Input: part model. Units: mm. Frame: model coordinates. A direction names the side the tool comes from. Round coordinates to 2 decimals unless told otherwise and drop trailing zeros. Loops run counter-clockwise (first coordinate to the right, second up) from the corner with the lowest first, then second, coordinate; pieces in that order, holes last. Notation, with made-up numbers: (44.25, 55) -> (55.25, 55) arc R8 ccw to (55.25, 69) -> close; hole circle Ø7 at (12.5, -0.5). An arc over 180 degrees is marked (long way). Answer in a Markdown table with one row per item. Add a question column.
Q1. Section D-D, the plane z = 2.75. Output: boundary loops of the cut face in (x, y), and give its area (3 significant figures).
Q2. Pin query (flat end, axial travel): pin 1 (5 mm diameter, centred on y = -7, z = 2.5, fed in from +X); pin 2 (1 mm diameter, centred on x = -5.5, y = -3, fed in from +Z); pin 3 (10 mm diameter, centred on x = 6, y = -4.5, fed in from -Z); pin 4 (0.5 mm diameter, centred on x = -5, z = 6.5, fed in from -Y). Return the tip coordinate at first contact, or that it passes through.
Q3. Section A-A, the plane z = 6.5. Output: boundary loops of the cut face in (x, y), and give its area (3 significant figures).
Q4. Ray query, L1, parallel to Y at x = 0, z = 11.1; L2, parallel to Y at x = 0, z = 10.25; L3, parallel to Y at x = 0, z = 11.75. Return the intervals inside material, ascending. Write a range as from..to.
Q5. Section B-B, the plane x = 0. Give the number of separate pieces and of enclosed holes in the cut face, and give its area (3 significant figures).
Q6. Reachability of faces 1 (the face through (-1, 8, 10.5)), 2 (the face through (0, 0, 11)), 3 (the face through (5.15, -8.98, 11.7)) from +Z, -Z, +X, -X, +Y, -Y: full face, straight path, thin tool, end or side. Return the list, or none.
Q7. Section C-C, the plane y = 0. Output: boundary loops of the cut face in (x, z), and give its area (3 significant figures).
Q8. Mould query, pull axis Y, two halves, no side actions, for faces 4 (the face through (0.05, -14.55, 10.75)), 5 (the face through (5.225, 8.869, 11.699)), 6 (the face through (-4.175, 0, 7)). Classes: pulls with the +Y half, pulls with the -Y half, needs draft (parallel to the pull), parting line crosses it, or undercut.
```python
from build123d import *

# Parameters (mm, degrees)
SKETCH1_R           = 7.5
BOSS_EXTRUDE1_DEPTH = 10.5
FILLET1_R           = 1
SKETCH2_R           = 6
BOSS_EXTRUDE2_DEPTH = 2
SKETCH3_R           = 1.6
BOSS_EXTRUDE3_DEPTH = 1.5
FILLET2_R           = 1
SKETCH4_R           = 7
CUT_EXTRUDE1_DEPTH  = 8.34
SKETCH5_R           = 5.8
BOSS_EXTRUDE4_DEPTH = 7.34
CUT_EXTRUDE2_START  = -7.34
CUT_EXTRUDE2_DEPTH  = 7.34


with BuildPart() as part:
    # Sketch1 → Boss-Extrude1 (new body)
    with BuildSketch(Plane.XY):
        with Locations(Location((0, 0, 0), (0, 0, 180))):
            Circle(SKETCH1_R)
    extrude(amount=BOSS_EXTRUDE1_DEPTH)

    # Fillet1
    fillet1_edges = [part.edges().sort_by_distance(p)[0] for p in [
        (7.5, 0, 0),
    ]]
    fillet(fillet1_edges, radius=FILLET1_R)

    # Sketch2 → Boss-Extrude2 (add)
    with BuildSketch(Plane(origin=(0, 0, 0), x_dir=(-1, 0, 0), z_dir=(0, 0, -1))):
        with Locations(Location((0, 0, 0), (0, 0, 180))):
            Circle(SKETCH2_R)
    extrude(amount=BOSS_EXTRUDE2_DEPTH)

    # Sketch3 → Boss-Extrude3 (add)
    with BuildSketch(Plane.XY.offset(10.5)):
        with BuildLine():
            Line((-7.964864241, 5.177927928), (-2.89250333, 12.980405405))
            ThreePointArc((-2.89250333, 12.980405405), (0, 14.55), (2.89250333, 12.980405405))
            Line((2.89250333, 12.980405405), (7.964864241, 5.177927928))
            ThreePointArc((7.964864241, 5.177927928), (9.5, 0), (7.964864241, -5.177927928))
            Line((7.964864241, -5.177927928), (2.89250333, -12.980405405))
            ThreePointArc((2.89250333, -12.980405405), (0, -14.55), (-2.89250333, -12.980405405))
            Line((-2.89250333, -12.980405405), (-7.964864241, -5.177927928))
            ThreePointArc((-7.964864241, -5.177927928), (-9.5, 0), (-7.964864241, 5.177927928))
        make_face()
        with Locations((0, -11.1)):
            Circle(SKETCH3_R, mode=Mode.SUBTRACT)
        with Locations((0, 11.1)):
            Circle(SKETCH3_R, mode=Mode.SUBTRACT)
    extrude(amount=BOSS_EXTRUDE3_DEPTH)

    # Fillet2
    fillet2_edges = [part.edges().sort_by_distance(p)[0] for p in [
        (-9.5, 0, 12),
        (-5.428683785, -9.079166667, 12),
        (0, -14.55, 12),
        (5.428683785, -9.079166667, 12),
        (9.5, 0, 12),
        (5.428683785, 9.079166667, 12),
        (0, 14.55, 12),
        (-5.428683785, 9.079166667, 12),
    ]]
    fillet(fillet2_edges, radius=FILLET2_R)

    # Sketch4 → Cut-Extrude1 (cut)
    with BuildSketch(Plane.XY.offset(12)):
        Circle(SKETCH4_R)
    extrude(amount=-CUT_EXTRUDE1_DEPTH, mode=Mode.SUBTRACT)

    # Sketch5 → Boss-Extrude4 (add)
    with BuildSketch(Plane.XY.offset(3.66)):
        with Locations(Location((0, 0, 0), (0, 0, 180))):
            Circle(SKETCH5_R)
    extrude(amount=BOSS_EXTRUDE4_DEPTH)

    # Sketch6 → Cut-Extrude2 (cut)
    with BuildSketch(Plane.XY.offset(11).offset(CUT_EXTRUDE2_START)):
        with BuildLine():
            Line((-5.674504384, -1.2), (-4.174504384, -1.2))
            Line((-4.174504384, -1.2), (-4.174504384, 1.2))
            Line((-4.174504384, 1.2), (-5.674504384, 1.2))
            ThreePointArc((-5.674504384, 1.2), (-5.8, 0), (-5.674504384, -1.2))
        make_face()
    extrude(amount=CUT_EXTRUDE2_DEPTH, mode=Mode.SUBTRACT)


solid = part.part
```
Answer block:
| question | item | result |
|---|---|---|
| 1 | outline | circle Ø15 at (0, 0) |
| 1 | area | 177 mm^2 |
| 2 | pin 1 | x = 6 |
| 2 | pin 2 | z = 11 |
| 2 | pin 3 | z = -2 |
| 2 | pin 4 | y = -5.8 |
| 3 | outline | circle Ø15 at (0, 0); (-5.67, -1.2) arc R5.8 ccw (long way) to (-5.67, 1.2) -> (-4.17, 1.2) -> (-4.17, -1.2) -> close; hole circle Ø14 at (0, 0) |
| 3 | area | 125 mm^2 |
| 4 | L1 | -14.54..-12.7, -9.5..-7, 7..9.5, 12.7..14.54 |
| 4 | L2 | -7.5..-7, -5.8..5.8, 7..7.5 |
| 4 | L3 | -14.21..-12.7, -9.5..-7, 7..9.5, 12.7..14.21 |
| 5 | separate pieces | 3 |
| 5 | enclosed holes | 0 |
| 5 | area | 183 mm^2 |
| 6 | face 1 | -Z |
| 6 | face 2 | +Z |
| 6 | face 3 | +Z, +X, -Y |
| 7 | outline | (-9.5, 10.5) -> (-7.5, 10.5) -> (-7.5, 1) arc R1 ccw to (-6.5, 0) -> (-6, 0) -> (-6, -2) -> (6, -2) -> (6, 0) -> (6.5, 0) arc R1 ccw to (7.5, 1) -> (7.5, 10.5) -> (9.5, 10.5) -> (9.5, 11) arc R1 ccw to (8.5, 12) -> (7, 12) -> (7, 3.66) -> (5.8, 3.66) -> (5.8, 11) -> (-4.17, 11) -> (-4.17, 3.66) -> (-7, 3.66) -> (-7, 12) -> (-8.5, 12) arc R1 ccw to (-9.5, 11) -> close |
| 7 | area | 166 mm^2 |
| 8 | face 4 | pulls with the -Y half |
| 8 | face 5 | pulls with the +Y half |
| 8 | face 6 | undercut |
